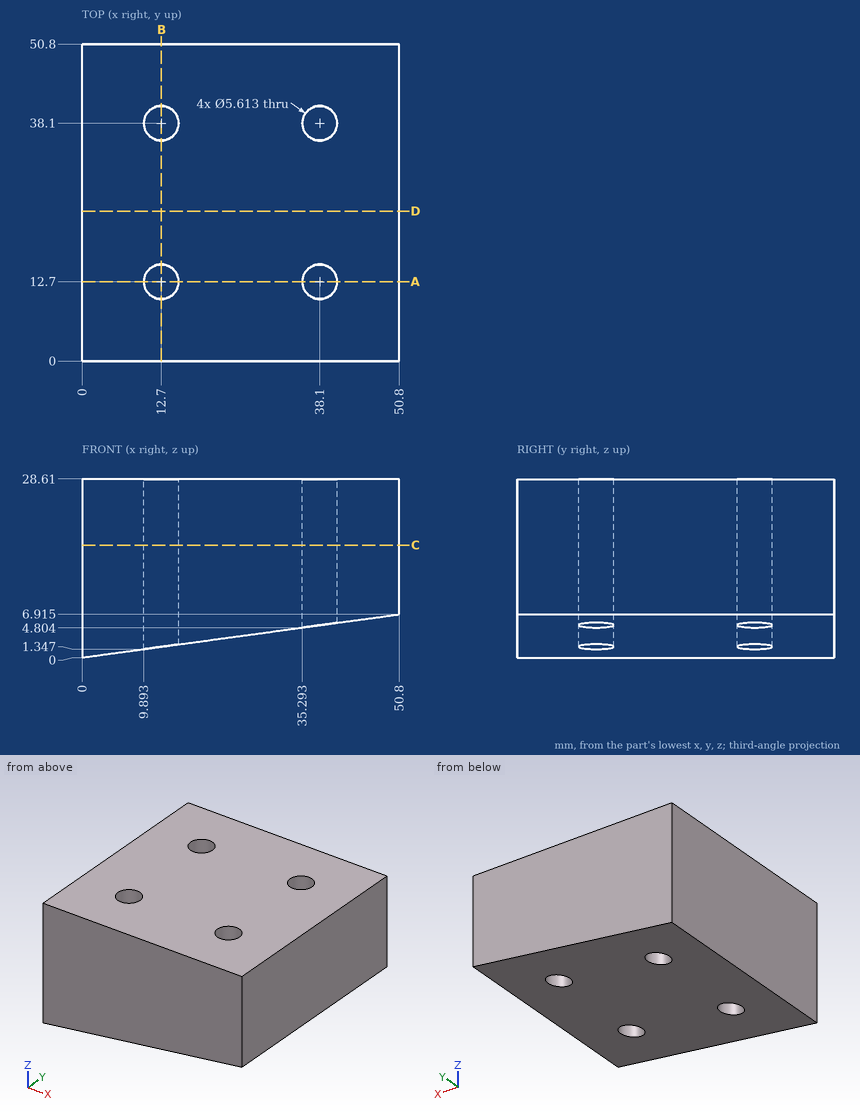
Verification items for this drawing (mm, ordinates from the low corner). Coordinates: 2 decimals unless noted, no trailing zeros. Order: outer loops, then holes, each group sorted by start corner. A loop starts at its lowest first (then second) coordinate and runs counter-clockwise, first axis right, second up. Notation, with made-up numbers: (0, -0.5) -> (49, -0.5) arc R13 ccw to (49, 23.5) -> close; hole circle Ø11 at (-12.5, 46.25). An arc over 180 degrees is marked (long way). Put each result on its own line as item: value. Start each with the question number.
1. Cross-section at A-A, the plane y = 12.7. Record the boundary of the cut face in (x, z) (1 decimal).
2. Material ranges on L1, parallel to Y at x = 38.1, z = 11.25; L2, parallel to Y at x = 12, z = 18.5, recorded low to high. Write a range as [from, to].
3. Cross-section at D-D, the plane y = 24. Record the boundary of the cut face in (x, z) (1 decimal).
4. Go/stop test with flat-tipped pins: pin 1 Ø9 at (x, y) = (12.7, 12.7) entering from -Z; pin 2 Ø8 at (y, z) = (37, 7.5) entering from -X; pin 3 Ø6.5 at (x, y) = (38.1, 38.1) entering from -Z; pin 4 Ø4 at (x, y) = (24.5, 44.5) entering from -Z. Record where each tip stops, or that it passes through.
5. Cross-section at C-C, the plane z = 18. Record the boundary of the cut face in (x, y), then the cut area to 3 significant figures.
6. Cross-section at B-B, the plane x = 12.7. Record the boundary of the cut face in (y, z).
Computed:
1. outline: (0, 0) -> (9.9, 1.3) -> (9.9, 28.6) -> (0, 28.6) -> close; (15.5, 2.1) -> (35.3, 4.8) -> (35.3, 28.6) -> (15.5, 28.6) -> close; (40.9, 5.6) -> (50.8, 6.9) -> (50.8, 28.6) -> (40.9, 28.6) -> close
2. L1: [0, 9.89], [15.51, 35.29], [40.91, 50.8]
2. L2: [0, 9.98], [15.42, 35.38], [40.82, 50.8]
3. outline: (0, 0) -> (50.8, 6.9) -> (50.8, 28.6) -> (0, 28.6) -> close
4. pin 1: z = 1.12
4. pin 2: x = 0
4. pin 3: z = 4.74
4. pin 4: z = 3.06
5. outline: (0, 0) -> (50.8, 0) -> (50.8, 50.8) -> (0, 50.8) -> close; hole circle Ø5.61 at (12.7, 12.7); hole circle Ø5.61 at (12.7, 38.1); hole circle Ø5.61 at (38.1, 12.7); hole circle Ø5.61 at (38.1, 38.1)
5. area: 2,480 mm2
6. outline: (0, 1.73) -> (9.89, 1.73) -> (9.89, 28.61) -> (0, 28.61) -> close; (15.51, 1.73) -> (35.29, 1.73) -> (35.29, 28.61) -> (15.51, 28.61) -> close; (40.91, 1.73) -> (50.8, 1.73) -> (50.8, 28.61) -> (40.91, 28.61) -> close
